Verification items for the finished model (mm, model axes). Round coordinates to 2 decimals unless told otherwise and drop trailing zeros. Write item = value, one per line.
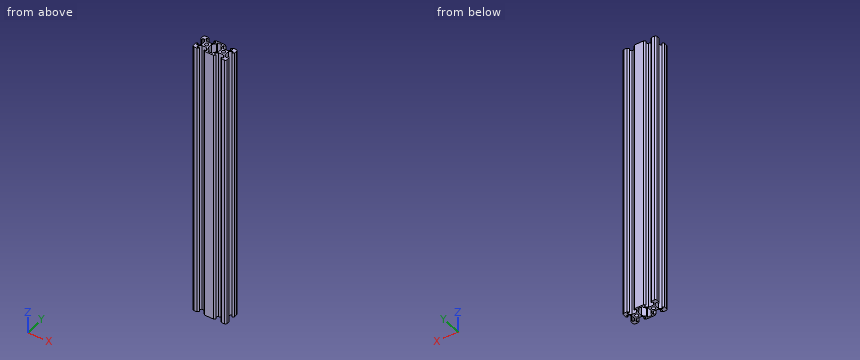
Autodesk Inventor part; units mm, degrees
ref_plane "Start Plane" through (0, 0, 10) normal (0, 0, 1) x (1, 0, 0)
ref_plane "End Plane" through (0, 0, 340) normal (0, 0, 1) x (1, 0, 0)
ref_plane "Work Plane6" through (-20, 4.5951, 340) normal (0, 0, 1) x (1, 0, 0)
ref_plane "Start Plane" through (0, 0, 10) normal (0, 0, 1) x (1, 0, 0)
ref_plane "End Plane" through (0, 0, 340) normal (0, 0, 1) x (1, 0, 0)
sketch "Sketch" plane through (0, 0, 0) normal (0, 0, 1) x (1, 0, 0)
  line L0 (0, 0) -> (0, 10) construction
  line L1 (-10, 10) -> (-10, 0) construction
  line L2 (0, 0) -> (-10, 0) construction
  circle A0 centre (-10, 0) radius 2.1
  line L3 (-13.9007, 3.9007) -> (-6.0993, 3.9007) construction
  line L4 (-6.0993, 3.9007) -> (-6.0993, -3.9007) construction
  line L5 (-6.0993, -3.9007) -> (-13.9007, -3.9007) construction
  line L6 (-13.9007, -3.9007) -> (-13.9007, 3.9007) construction
  line L7 (-13.9007, 3.9007) -> (-6.0993, -3.9007) construction
  line L8 (-6.0993, 3.9007) -> (-13.9007, -3.9007) construction
  line L9 (-13.9007, -2.84) -> (-12.84, -3.9007) construction
  line L10 (-13.9007, -2.84) -> (-12.4007, -2.84) construction
  line L11 (-12.84, -3.9007) -> (-15.4993, -6.56)
  line L12 (-15.4993, -6.56) -> (-15.4993, -8.2)
  line L13 (-15.4993, -8.2) -> (-12.84, -8.2)
  line L14 (-12.84, -8.2) -> (-14.64, -10)
  line L15 (-7.16, -3.9007) -> (-4.5007, -6.56)
  line L16 (-4.5007, -6.56) -> (-4.5007, -8.2)
  line L17 (-4.5007, -8.2) -> (-7.16, -8.2)
  line L18 (-7.16, -8.2) -> (-5.36, -10)
  line L19 (-12.84, -3.9007) -> (-7.16, -3.9007)
  line L20 (-12.84, 3.9007) -> (-13.9007, 2.84) construction
  line L21 (-12.84, 3.9007) -> (-12.84, 2.4007) construction
  line L22 (-13.9007, 2.84) -> (-16.56, 5.4993)
  line L23 (-16.56, 5.4993) -> (-18.2, 5.4993)
  line L24 (-18.2, 5.4993) -> (-18.2, 2.84)
  line L25 (-18.2, 2.84) -> (-20, 4.64)
  line L26 (-18.2, -2.84) -> (-20, -4.64)
  line L27 (-18.2, -5.4993) -> (-18.2, -2.84)
  line L28 (-16.56, -5.4993) -> (-18.2, -5.4993)
  line L29 (-13.9007, -2.84) -> (-16.56, -5.4993)
  line L30 (-13.9007, 2.84) -> (-13.9007, -2.84)
  line L31 (-6.0993, 2.84) -> (-7.16, 3.9007) construction
  line L32 (-6.0993, 2.84) -> (-7.5993, 2.84) construction
  line L33 (-7.16, 3.9007) -> (-4.5007, 6.56)
  line L34 (-4.5007, 6.56) -> (-4.5007, 8.2)
  line L35 (-4.5007, 8.2) -> (-7.16, 8.2)
  line L36 (-7.16, 8.2) -> (-5.36, 10)
  line L37 (-12.84, 8.2) -> (-14.64, 10)
  line L38 (-15.4993, 8.2) -> (-12.84, 8.2)
  line L39 (-15.4993, 6.56) -> (-15.4993, 8.2)
  line L40 (-12.84, 3.9007) -> (-15.4993, 6.56)
  line L41 (-7.16, 3.9007) -> (-12.84, 3.9007)
  line L42 (-6.0993, 2.84) -> (-2.6993, 6.24)
  line L43 (-2.6993, 6.24) -> (-2.6993, 8.2)
  line L44 (-4.5007, 8.2) -> (0, 8.2) construction
  line L45 (-6.0993, -2.84) -> (-2.6993, -6.24)
  line L46 (-2.6993, -6.24) -> (-2.6993, -8.2)
  line L47 (10, 10) -> (10, 0) construction
  circle A1 centre (10, 0) radius 2.1
  line L48 (13.9007, 3.9007) -> (6.0993, -3.9007) construction
  line L49 (13.9007, -2.84) -> (12.84, -3.9007) construction
  line L50 (12.84, -3.9007) -> (15.4993, -6.56)
  line L51 (15.4993, -6.56) -> (15.4993, -8.2)
  line L52 (15.4993, -8.2) -> (12.84, -8.2)
  line L53 (12.84, -8.2) -> (14.64, -10)
  line L54 (7.16, -8.2) -> (5.36, -10)
  line L55 (4.5007, -8.2) -> (7.16, -8.2)
  line L56 (4.5007, -6.56) -> (4.5007, -8.2)
  line L57 (7.16, -3.9007) -> (4.5007, -6.56)
  line L58 (12.84, -3.9007) -> (7.16, -3.9007)
  line L59 (13.9007, 2.84) -> (13.9007, -2.84)
  line L60 (13.9007, 2.84) -> (16.56, 5.4993)
  line L61 (16.56, 5.4993) -> (18.2, 5.4993)
  line L62 (18.2, 5.4993) -> (18.2, 2.84)
  line L63 (18.2, 2.84) -> (20, 4.64)
  line L64 (18.2, -5.4993) -> (18.2, -2.84)
  line L65 (18.2, -2.84) -> (20, -4.64)
  line L66 (16.56, -5.4993) -> (18.2, -5.4993)
  line L67 (13.9007, -2.84) -> (16.56, -5.4993)
  line L68 (7.16, 3.9007) -> (12.84, 3.9007)
  line L69 (7.16, 3.9007) -> (4.5007, 6.56)
  line L70 (4.5007, 6.56) -> (4.5007, 8.2)
  line L71 (4.5007, 8.2) -> (7.16, 8.2)
  line L72 (7.16, 8.2) -> (5.36, 10)
  line L73 (15.4993, 8.2) -> (12.84, 8.2)
  line L74 (12.84, 8.2) -> (14.64, 10)
  line L75 (15.4993, 6.56) -> (15.4993, 8.2)
  line L76 (12.84, 3.9007) -> (15.4993, 6.56)
  line L77 (6.0993, 2.84) -> (2.6993, 6.24)
  line L78 (2.6993, 6.24) -> (2.6993, 8.2)
  line L79 (6.0993, -2.84) -> (2.6993, -6.24)
  line L80 (2.6993, -6.24) -> (2.6993, -8.2)
  line L81 (-14.64, -10) -> (-18.2, -10)
  line L82 (-20, -8.2) -> (-20, -4.64)
  line L83 (-20, 4.64) -> (-20, 8.2)
  line L84 (-18.2, 10) -> (-14.64, 10)
  line L85 (18.2, -10) -> (14.64, -10)
  line L86 (5.36, -10) -> (-5.36, -10)
  line L87 (-5.36, 10) -> (5.36, 10)
  line L88 (14.64, 10) -> (18.2, 10)
  line L89 (20, 8.2) -> (20, 4.64)
  line L90 (20, -4.64) -> (20, -8.2)
  line L91 (-2.6993, -8.2) -> (2.6993, -8.2)
  line L92 (-2.6993, 8.2) -> (2.6993, 8.2)
  line L93 (-6.0993, 2.84) -> (-6.0993, -2.84)
  line L94 (6.0993, 2.84) -> (6.0993, -2.84)
  arc A2 (-20, -8.2) -> (-18.2, -10) centre (-18.2, -8.2) ccw
  arc A3 (-18.2, 10) -> (-20, 8.2) centre (-18.2, 8.2) ccw
  arc A4 (18.2, -10) -> (20, -8.2) centre (18.2, -8.2) ccw
  arc A5 (20, 8.2) -> (18.2, 10) centre (18.2, 8.2) ccw
  point P0 (-13.9007, -3.9007)
  point P1 (-13.9007, 3.9007)
  point P2 (-13.9007, 3.9007)
  point P3 (-6.0993, 3.9007)
  point P4 (6.0993, 3.9007)
  point P5 (13.9007, -3.9007)
  point P6 (12.4007, -2.84)
  point P7 (13.9007, -3.9007)
  point P8 (13.9007, 3.9007)
  point P9 (12.84, 3.9007)
  point P10 (12.84, 2.4007)
  point P11 (13.9007, 3.9007)
  point P12 (6.0993, 3.9007)
  point P13 (7.5993, 2.84)
  point P14 (-20, 10)
  point P15 (20, -10)
  point P16 (20, 10)
  point P17 (-20, -10)
  dimension "d26" = 10
  dimension "d27" = 10
  dimension "d28" = 4.2
  dimension "d29" = 1.5
  dimension "d30" = 45
  dimension "d32" = 45
  dimension "d33" = 1.64
  dimension "d34" = 1.8
  dimension "d35" = 10
  dimension "d36" = 5.68
  dimension "d39" = 180
  dimension "d41" = 1.96
  dimension "d42" = 5.68
  dimension "d45" = 1.8
extrude "Body" add sketch "Sketch" along normal up to surface (330 mm away) from surface at 10
sketch "Sketch8" plane through (0, 0, 0) normal (0, 0, 1) x (1, 0, 0)
  line L0 (0, 0) -> (10, 0)
ref_plane "Work Plane5" through (0, 0, 0) normal (0, -1, 0) x (1, 0, 0)
sketch "Sketch9" plane through (0, 0, 0) normal (0, -1, 0) x (1, 0, 0)
  line L0 (-2, 10) -> (12, 10)
  line L1 (-2, 340) -> (12, 340)
  dimension "d51" = 330
ref_plane "Work Plane6" through (-20, 4.5951, 340) normal (0, 0, 1) x (1, 0, 0)
split "Split1" plane through (-20, 4.5951, 340) removes the side toward (0, 0, 1)
ref_plane "Work Plane7" through (255, 4.5951, 10) normal (0, 0, -1) x (-1, 0, 0)
split "Split2" plane through (255, 4.5951, 10) removes the side toward (0, 0, -1)
equation "\"d42\" = d36"
equation "\"G_L\" = d51"
properties part number "vslot 20 x 40" material "Aluminum 6061"
(1) Go/stop test with flat-tipped pins: pin 1 Ø4.5 at (y, z) = (-0.5, 210) entering from +X; pin 2 Ø1.3 at (x, z) = (-14.5, 114) entering from +Y; pin 3 Ø1.7 at (x, z) = (10.5, 256) entering from +Y; pin 4 Ø2 at (x, z) = (6.5, 157.5) entering from -Y. Record where each tip stops, or that it passes through.
Filled sheet:
pin_1 = 13.9
pin_2 = 10
pin_3 = 3.9
pin_4 = -9.86
(2) Material ranges on probe 1 along X at (y, z) = (0.25, 185); probe 2 along X at (y, z) = (7.75, 29); probe 3 along Y at (x, z) = (-10, 192), recorded low to high. Write a range as from..to.
Filled sheet:
probe_1 = -13.9..-12.09, -7.91..-6.1, 6.1..7.91, 12.09..13.9
probe_2 = -20..-15.5, -4.5..-2.7, 2.7..4.5, 15.5..20
probe_3 = -3.9..-2.1, 2.1..3.9
(3) Sectioned sample at A-A, the plane z = 226. Count the separate pieces of the cut face and the enclosed holes in it, and give its area (3 significant figures).
Filled sheet:
separate_pieces = 1
enclosed_holes = 3
area = 297 mm2
